```python
from build123d import *

# Parameters (mm, degrees)
F0_W     = 375
F0_H     = 100
F1_DEPTH = 50
F2_R     = 5
F3_DEPTH = 75
F4_W     = 100
F4_H     = 50
F5_DEPTH = 50.001
F6_R     = 5
F7_DEPTH = 50.001
F8_R     = 5
F9_DEPTH = 25


with BuildPart() as f1:
    # F0 (on Front) → F1 (new body)
    with BuildSketch(Plane.XZ):
        Rectangle(F0_W, F0_H)
    extrude(amount=F1_DEPTH)

    # F2 (on face) → F3 (cut)
    with BuildSketch(Plane.XY.offset(50)):
        with Locations((97.5, -25)):
            Circle(F2_R)
        with Locations((177.5, -25)):
            Circle(F2_R)
    extrude(amount=-F3_DEPTH, mode=Mode.SUBTRACT)

    # F4 (on face) → F5 (cut, through all)
    with BuildSketch(Plane.XZ.offset(50)):
        with Locations((137.5, 25)):
            Rectangle(F4_W, F4_H)
    extrude(amount=-F5_DEPTH, mode=Mode.SUBTRACT)

    # F6 (on face) → F7 (cut, through all)
    with BuildSketch(Plane(origin=(0, 0, 0), x_dir=(-1, 0, 0), z_dir=(0, 1, 0))):
        with Locations((-112.5, -25)):
            Circle(F6_R)
        with Locations((-162.5, -25)):
            Circle(F6_R)
        with Locations((162.5, 25)):
            Circle(F6_R)
        with Locations((112.5, 25)):
            Circle(F6_R)
    extrude(amount=-F7_DEPTH, mode=Mode.SUBTRACT)

    # F8 (on face) → F9 (cut)
    with BuildSketch(Plane(origin=(0, 0, -50), x_dir=(1, 0, 0), z_dir=(0, 0, -1))):
        with Locations((-162.5, 25)):
            Circle(F8_R)
        with Locations((-112.5, 25)):
            Circle(F8_R)
    extrude(amount=-F9_DEPTH, mode=Mode.SUBTRACT)


solid = f1.part
```
Geometry check sheet. Reference: the model listing, model coordinates, mm. A direction names the side the tool comes from. Coordinates: 2 decimals unless noted, no trailing zeros. Order: outer loops, then holes, each group sorted by start corner. A loop starts at its lowest first (then second) coordinate and runs counter-clockwise, first axis right, second up. Notation, with made-up numbers: (68.5, -32.75) - (127.5, -32.75) arc R10 ccw to (127.5, -28.75) - close; hole circle Ø1 at (-14.75, 52.5). An arc over 180 degrees is marked (long way). Answer in a Markdown table with one row per item. Add a question column.
1. Section check C-C (x = 162.5). Enter the section's corners in (y, z), plus the area to 3 significant figures.
2. Section check B-B (y = -34.5). Enter the section's corners in (x, z), plus the area to 3 significant figures.
3. Material ranges on L1, parallel to X at y = -25, z = -41; L2, parallel to Z at x = 162.5, y = -11.5; L3, parallel to Z at x = -112, y = -22, recorded low to high. Write a range as [from, to].
4. Section check A-A (x = -112.5). Enter the section's corners in (y, z).
5. Access from +Z, -Z, +X, -X, +Y, -Y to the whole of each face (thin tool, end or side, straight path). Record for faces 5 (the face through (166.5, -24.6, -28)), 6 (the face through (-163, -25, -25)), 7 (the face through (137, -25, 0)), 8 (the face through (97, -25, -25)).
6. Draft check along Y on faces 1 (the face through (-110.193, -20.564, -37.675)), 2 (the face through (-44, -50, 1)), 3 (the face through (-44, 0, 1)), 4 (the face through (-52, -25, 50)). Enter one of: +Y half, -Y half, draft (parallel to the pull), parting line (faces both ways), or undercut.
7. Gauge pin test, flat ends, axial feed: pin 1 Ø6 at (x, y) = (-112.5, -25) entering from -Z; pin 2 Ø16 at (x, y) = (177.5, -25) entering from +Z; pin 3 Ø25 at (y, z) = (-30.5, 35) entering from +X. Record the tip position at first contact, or that the pin passes through.
Data:
| question | item | result |
|---|---|---|
| 1 | outline | (-50, -50) - (0, -50) - (0, -30) - (-50, -30) - close; (-50, -20) - (0, -20) - (0, 0) - (-50, 0) - close |
| 1 | area | 2,000 mm² |
| 2 | outline | (-187.5, -50) - (187.5, -50) - (187.5, 0) - (87.5, 0) - (87.5, 50) - (-187.5, 50) - close; hole circle Ø10 at (-162.5, 25); hole circle Ø10 at (-112.5, 25); hole circle Ø10 at (112.5, -25); hole circle Ø10 at (162.5, -25) |
| 2 | area | 32,200 mm² |
| 3 | L1 | x = [-187.5, -167.5], [-157.5, -117.5], [-107.5, 187.5] |
| 3 | L2 | z = [-50, -30], [-20, 0] |
| 3 | L3 | z = [-25, 20.03], [29.97, 50] |
| 4 | outline | (-50, -50) - (-30, -50) - (-30, -25) - (-20, -25) - (-20, -50) - (0, -50) - (0, 20) - (-50, 20) - close; (-50, 30) - (0, 30) - (0, 50) - (-50, 50) - close |
| 5 | face 5 | +Y, -Y |
| 5 | face 6 | -Z |
| 5 | face 7 | +Z, +X, +Y, -Y |
| 5 | face 8 | +Z |
| 6 | face 1 | undercut |
| 6 | face 2 | -Y half |
| 6 | face 3 | +Y half |
| 6 | face 4 | draft |
| 7 | pin 1 | stops at z = -25 |
| 7 | pin 2 | stops at z = 0 |
| 7 | pin 3 | stops at x = 87.5 |
